Answer from the drawing. Dimensions are ordinates in mm from the lowest x, y and z of the part. Round coordinates to 2 decimals unless told otherwise and drop trailing zeros. Loops run counter-clockwise (first coordinate to the right, second up) from the corner with the lowest first, then second, coordinate; pieces in that order, holes last. Notation, with made-up numbers: (-33, 45.25) - (-21, 45.25) arc R11 ccw to (-21, 49.25) - close; hole circle Ø1 at (80, 83). An arc over 180 degrees is marked (long way). Answer as CSV lines item,"result".
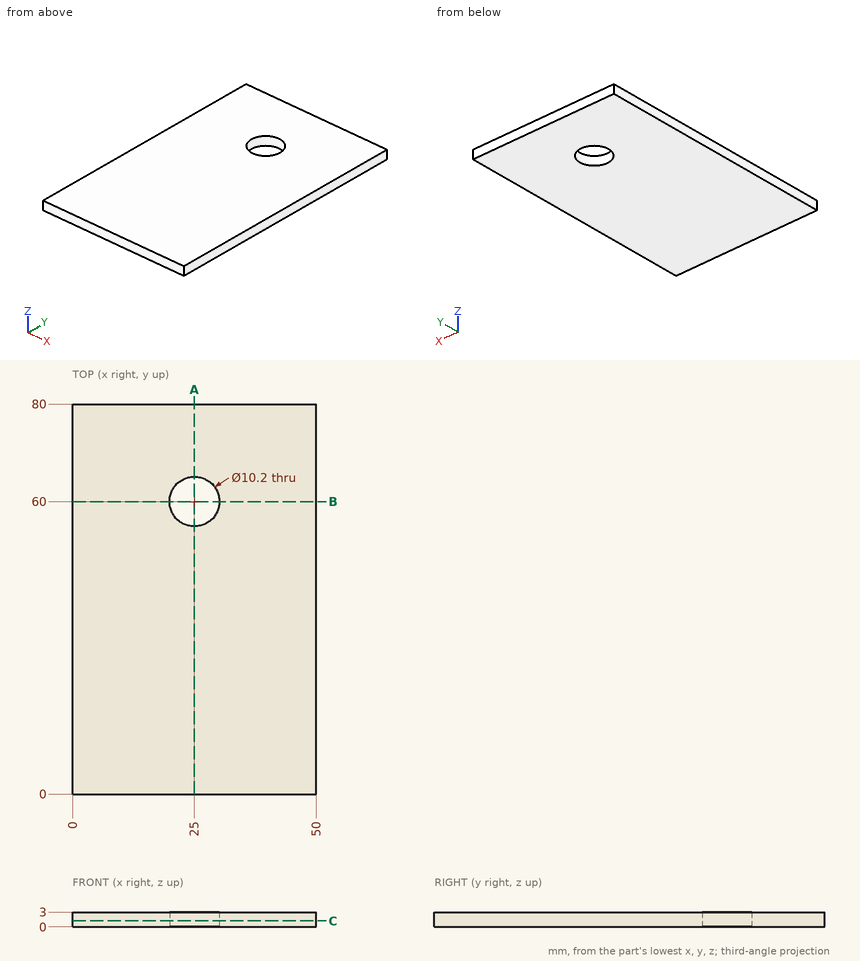
1) A cutting plane is placed at A-A, the plane x = 25. Determine the outline of the cut face in (y, z).
Entries:
outline,"(0, 0) - (54.9, 0) - (54.9, 3) - (0, 3) - close; (65.1, 0) - (80, 0) - (80, 3) - (65.1, 3) - close"
2) A cutting plane is placed at B-B, the plane y = 60. Determine the outline of the cut face in (x, z).
Entries:
outline,"(0, 0) - (19.9, 0) - (19.9, 3) - (0, 3) - close; (30.1, 0) - (50, 0) - (50, 3) - (30.1, 3) - close"
3) Find the intervals of material crossed by line 1 (Y direction, x = 25, z = 0.85), in increasing order.
Entries:
line 1,"y = 0 to 54.9, 65.1 to 80"
4) A cutting plane is placed at C-C, the plane z = 1.2. Determine the outline of the cut face in (x, y).
Entries:
outline,"(0, 0) - (50, 0) - (50, 80) - (0, 80) - close; hole circle Ø10.2 at (25, 60)"
5) This flat-tipped pin is pushed along its axis until it touches: P1, Ø1, axis at y = 31, z = 0.5, coming from the -X side. Where does it stop, or does it pass through?
Entries:
P1,"stops at x = 0"
